For this review, take the finished solid that the model builds, in its own axes (mm). Round coordinates to 2 decimals unless told otherwise and drop trailing zeros. Write each loop counter-clockwise with the first axis right and the second up, starting at its lowest first coordinate (ties: lowest second). Pieces come first, ordered by that corner, then holes. Notation, with made-up numbers: (59, -18.75) - (91, -18.75) arc R18 cw to (91, -8.75) - close; hole circle Ø3 at (-5.5, -4.75). An arc over 180 degrees is marked (long way). Answer in a Markdown table with one row per item. Add a question column.
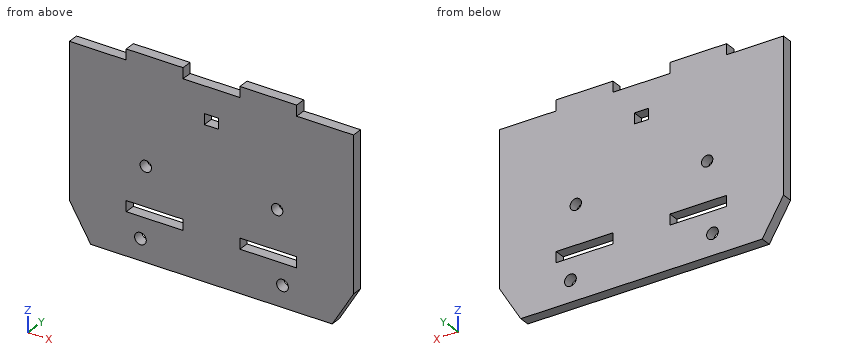
from build123d import *

# Parameters (mm, degrees)
SKETCH1_R           = 1.65
BOSS_EXTRUDE1_DEPTH = 3
SKETCH2_R           = 1.6
SKETCH2_W           = 4
SKETCH2_H           = 3
SKETCH2_W_2         = 16
CUT_EXTRUDE1_DEPTH  = 4


with BuildPart() as part:
    # Sketch1 → Boss-Extrude1 (new body)
    with BuildSketch(Plane(origin=(0, 0, 0), x_dir=(1, 0, 0), z_dir=(0, 1, 0))):
        Polygon((-40, 37), (-34, 47), (34, 47), (40, 37), (40, -6), (24, -6), (24, -9), (8, -9), (8, -6), (-8, -6), (-8, -9), (-24, -9), (-24, -6), (-40, -6), align=None)
        with Locations((-20, 41)):
            Circle(SKETCH1_R, mode=Mode.SUBTRACT)
        with Locations((20, 41.003103662)):
            Circle(SKETCH1_R, mode=Mode.SUBTRACT)
    extrude(amount=BOSS_EXTRUDE1_DEPTH)

    # Sketch2 → Cut-Extrude1 (cut, through all)
    with BuildSketch(Plane(origin=(0, 3, 0), x_dir=(1, 0, 0), z_dir=(0, 1, 0))):
        with Locations((-18.5, 21)):
            Circle(SKETCH2_R)
        with Locations((18.5, 21)):
            Circle(SKETCH2_R)
        with Locations((0, 3)):
            Rectangle(SKETCH2_W, SKETCH2_H)
        with Locations((-16, 33.5)):
            Rectangle(SKETCH2_W_2, SKETCH2_H)
        with Locations((16, 33.5)):
            Rectangle(SKETCH2_W_2, SKETCH2_H)
    extrude(amount=-CUT_EXTRUDE1_DEPTH, mode=Mode.SUBTRACT)


solid = part.part
Q1. Insertion check: pin 1 Ø1.9 at (x, z) = (-18.5, -21) entering from -Y (3 decimals); pin 2 Ø3 at (x, z) = (-4, -34.5) entering from -Y; pin 3 Ø1.5 at (y, z) = (1.5, 7) entering from -X; pin 4 Ø0.9 at (x, y) = (2, 1.5) entering from +Z. Each pin has a flat end and moves straight along its axis. Give the tip position at first contact, or say it passes through.
Q2. Add section B-B on x = 22.5. State the section outline as (y, z) points, then the cut area to 3 significant figures.
Q3. Add section A-A on z = -21. State the section outline as (x, y) points.
Q4. To check wall thickness, follow probe 1 along X at (y, z) = (1.65, -21); probe 2 along X at (y, z) = (1.15, -34); probe 3 along Z at (x, y) = (-17.5, 0.9). State the ranges of each line that lie inside material, in increasing order.
Answer sheet:
| question | item | result |
|---|---|---|
| 1 | pin 1 | passes through |
| 1 | pin 2 | stops at y = 0 |
| 1 | pin 3 | stops at x = -24 |
| 1 | pin 4 | stops at z = 6 |
| 2 | outline | (0, -47) - (3, -47) - (3, -35) - (0, -35) - close; (0, -32) - (3, -32) - (3, 9) - (0, 9) - close |
| 2 | area | 159 mm² |
| 3 | outline | (-40, 0) - (-20.1, 0) - (-20.1, 3) - (-40, 3) - close; (-16.9, 0) - (16.9, 0) - (16.9, 3) - (-16.9, 3) - close; (20.1, 0) - (40, 0) - (40, 3) - (20.1, 3) - close |
| 4 | probe 1 | x = -40 to -20.1, -16.9 to 16.9, 20.1 to 40 |
| 4 | probe 2 | x = -40 to -24, -8 to 8, 24 to 40 |
| 4 | probe 3 | z = -47 to -35, -32 to -22.25, -19.75 to 9 |
